The listing builds one solid part. Answer for the finished solid, in the listing's coordinates (mm). A direction names the side the tool comes from. Round coordinates to 2 decimals unless told otherwise and drop trailing zeros. Write each loop counter-clockwise with the first axis right and the second up, starting at its lowest first coordinate (ties: lowest second). Pieces come first, ordered by that corner, then holes. Notation, with made-up numbers: (-2.5, 55.5) - (17.5, 55.5) arc R21 ccw to (17.5, 84.5) - close; hole circle Ø9 at (-11, 52.5). An arc over 180 degrees is marked (long way). Answer in a Markdown table with one row per item.
from build123d import *

# Parameters (mm, degrees)
SKETCH4_R          = 0.9921875
CUT_EXTRUDE1_DEPTH = 1.016
SKETCH3_R          = 0.9921875
CUT_EXTRUDE2_DEPTH = 2.54
FILLET1_R          = 0.635
FILLET1_2_R        = 1.5875
FILLET1_3_R        = 0.381


with BuildPart() as part:
    # Sketch2 → Revolve1 (revolve)
    with BuildSketch(Plane(origin=(0, 0, 0), x_dir=(0, 0, -1), z_dir=(1, 0, 0))):
        with BuildLine():
            Line((-1.27, 0.9921875), (-1.27, 0))
            Line((-1.27, 0), (9.525, 0))
            Line((9.525, 0), (12.7, 0))
            Line((12.7, 0), (12.7, 3.4925))
            Line((12.7, 3.4925), (9.525, 3.4925))
            Line((9.525, 3.4925), (9.525, 2.38125))
            Line((9.525, 2.38125), (0, 2.38125))
            Line((0, 2.38125), (0, 4.6228))
            Line((0, 4.6228), (-0.1778, 4.6228))
            ThreePointArc((-0.1778, 4.6228), (-0.991036966, 2.887856773), (-1.27, 0.9921875))
        make_face()
    revolve(axis=Axis((0, 0, 7.600580616), (0, 0, 1)))

    # Sketch4 → Cut-Extrude1 (cut)
    with BuildSketch(Plane.XY.offset(1.27)):
        Circle(SKETCH4_R)
    extrude(amount=-CUT_EXTRUDE1_DEPTH, mode=Mode.SUBTRACT)

    # Sketch3 → Cut-Extrude2 (cut)
    with BuildSketch(Plane(origin=(0, 0, -12.7), x_dir=(-1, 0, 0), z_dir=(0, 0, -1))):
        Circle(SKETCH3_R)
    extrude(amount=-CUT_EXTRUDE2_DEPTH, mode=Mode.SUBTRACT)

    # Fillet1
    fillet1_edges = [part.edges().sort_by_distance(p)[0] for p in [
        (0, -3.4925, -9.525),
    ]]
    fillet(fillet1_edges, radius=FILLET1_R)

    # Fillet1 2
    fillet1_2_edges = [part.edges().sort_by_distance(p)[0] for p in [
        (0, -3.4925, -12.7),
    ]]
    fillet(fillet1_2_edges, radius=FILLET1_2_R)

    # Fillet1 3
    fillet1_3_edges = [part.edges().sort_by_distance(p)[0] for p in [
        (0, -2.38125, 0),
        (-0.701582509, -0.701582509, 1.27),
        (-0.9921875, 0, 0.254),
    ]]
    fillet(fillet1_3_edges, radius=FILLET1_3_R)


solid = part.part
(1) For a pull along X with two mould halves and no side action, classify faces 1 (the cylindrical face through (1.45, -1.89, -4.89)), 2 (the flat face through (3, 0, 0)), 3 (the cylindrical face through (0.215, -0.969, -11.448)) as pulls with the +X half, pulls with the -X half, needs draft (parallel to the pull), parting line crosses it, or undercut.
Checked values:
| item | result |
|---|---|
| face 1 | parting line crosses it |
| face 2 | needs draft |
| face 3 | undercut |
(2) Section A-A (z = -10.5) is taken. Give the vertices of the cut face in (x, y) (1 decimal), and give its area (3 significant figures).
Checked values:
| item | result |
|---|---|
| outline | circle Ø7 at (0, 0); hole circle Ø2 at (0, 0) |
| area | 35.2 mm2 |
(3) For faces 4 (the flat face through (0, 0, 0.254)), 5 (the flat face through (1, -1, -12.7)), 6 (the cylindrical face through (-3.463, -0.455, -10.63)), determine the directions among +Z, -Z, +X, -X, +Y, -Y from which every point of the face is accessible in a straight line to the end or side of a thin tool.
Checked values:
| item | result |
|---|---|
| face 4 | +Z |
| face 5 | -Z, +X, -X, +Y, -Y |
| face 6 | -Z |
(4) Section B-B (z = -6.5) is taken. Give the vertices of the cut face in (x, y).
Checked values:
| item | result |
|---|---|
| outline | circle Ø4.76 at (0, 0) |
(5) Flat-ended cylindrical pins translate along their axes: pin 1 (4 mm diameter, centred on y = -2, z = -1, fed in from -X) (3 decimals); pin 2 (4 mm diameter, centred on x = 2.5, z = -6.5, fed in from +Y); pin 3 (3 mm diameter, centred on y = 2, z = -1, fed in from -X); pin 4 (4 mm diameter, centred on x = 2.5, y = 3, fed in from -Z). Find the tip coordinate at first contact, or state that the pin passes through.
Checked values:
| item | result |
|---|---|
| pin 1 | stops at x = -4.615 |
| pin 2 | stops at y = 2.33 |
| pin 3 | stops at x = -4.54 |
| pin 4 | stops at z = -12.7 |
(6) Find the intervals of material crossed by line 1 (Y direction, x = 0, z = -11.1); line 2 (Y direction, x = 0, z = 0.75); line 3 (X direction, y = 0, z = 0.7), in increasing order.
Checked values:
| item | result |
|---|---|
| line 1 | y = -3.49 to -0.99, 0.99 to 3.49 |
| line 2 | y = -3.56 to -0.99, 0.99 to 3.56 |
| line 3 | x = -3.67 to -0.99, 0.99 to 3.67 |
